Source: CAD feature listing. Evaluate the final solid. Frame: model axes, mm. Face numbers are marked on the shaded views. Round coordinates to 2 decimals unless told otherwise and drop trailing zeros. Order: outer loops, then holes, each group sorted by start corner. A loop starts at its lowest first (then second) coordinate and runs counter-clockwise, first axis right, second up. Notation, with made-up numbers: M -6,28 L 50,28 A25 cw 50,41 Z; hole C 50,-7.75 d7. An arc over 180 degrees is marked long. Use one line per item in the form item = value. Start each with the question number.
Q1. Section A-A (x = 29.8). Give the number of separate pieces and of enclosed holes in the cut face, plus the area to 3 significant figures.
Q2. Section D-D (x = 25.5). Return the cut outline in (y, z), plus the area to 3 significant figures.
Q3. Pull-direction query (Y, two-part tool) for the marked faces 1, 2 and 3; classes: pulls with the +Y half, pulls with the -Y half, needs draft (parallel to the pull), parting line crosses it, or undercut.
Q4. Section C-C (z = 7). Return the cut outline in (x, y).
Q5. Contact query for flat-ended pins moving along their axis: pin 1 (4.5 mm diameter, centred on x = 29.8, y = 9.8, fed in from +Z); pin 2 (5 mm diameter, centred on x = 30, y = 10.5, fed in from +Z); pin 3 (6 mm diameter, centred on x = 35, y = 12, fed in from +Z). Output: stop coordinate, or through.
Q6. Material intervals for probe 1 along Y at (x, z) = (9.8, 4.25); probe 2 along Y at (x, z) = (29.8, 0.85); probe 3 along Y at (x, z) = (5.5, 8), sorted ascending.
from build123d import *

# Parameters (mm, degrees)
SKETCH_W        = 39.6
SKETCH_H        = 39.6
PAD_DEPTH       = 9
SKETCH001_R     = 1.75
POCKET_DEPTH    = 10
SKETCH002_R     = 3
POCKET001_DEPTH = 6
SKETCH003_W     = 30
SKETCH003_H     = 30
POCKET002_DEPTH = 3
FILLET_R        = 1


with BuildPart() as part:
    # Sketch → Pad (new body)
    with BuildSketch(Plane.XY):
        with Locations((19.8, 19.8)):
            Rectangle(SKETCH_W, SKETCH_H)
    extrude(amount=PAD_DEPTH)

    # Sketch001 → Pocket (cut)
    with BuildSketch(Plane.XY.offset(9)):
        with Locations((9.8, 9.8)):
            Circle(SKETCH001_R)
        with Locations((9.8, 29.8)):
            Circle(SKETCH001_R)
        with Locations((29.8, 9.8)):
            Circle(SKETCH001_R)
        with Locations((29.8, 29.8)):
            Circle(SKETCH001_R)
    extrude(amount=-POCKET_DEPTH, mode=Mode.SUBTRACT)

    # Sketch002 → Pocket001 (cut)
    with BuildSketch(Plane.XY.offset(9)):
        with Locations((9.8, 9.8)):
            Circle(SKETCH002_R)
        with Locations((9.8, 29.8)):
            Circle(SKETCH002_R)
        with Locations((29.8, 9.8)):
            Circle(SKETCH002_R)
        with Locations((29.8, 29.8)):
            Circle(SKETCH002_R)
    extrude(amount=-POCKET001_DEPTH, mode=Mode.SUBTRACT)

    # Sketch003 → Pocket002 (cut)
    with BuildSketch(Plane.XY.offset(9)):
        with Locations((19.8, 19.8)):
            Rectangle(SKETCH003_W, SKETCH003_H)
    extrude(amount=-POCKET002_DEPTH, mode=Mode.SUBTRACT)

    # Fillet
    fillet_edges = [part.edges().sort_by_distance(p)[0] for p in [
        (0, 39.6, 4.5),
        (0, 0, 4.5),
        (39.6, 39.6, 4.5),
        (39.6, 0, 4.5),
        (39.6, 19.8, 0),
        (19.8, 39.6, 0),
        (0, 19.8, 0),
        (19.8, 0, 0),
        (19.8, 0, 9),
        (39.6, 19.8, 9),
        (19.8, 39.6, 9),
        (0, 19.8, 9),
        (19.8, 4.8, 9),
        (34.8, 19.8, 9),
        (19.8, 34.8, 9),
        (4.8, 19.8, 9),
    ]]
    fillet(fillet_edges, radius=FILLET_R)


solid = part.part
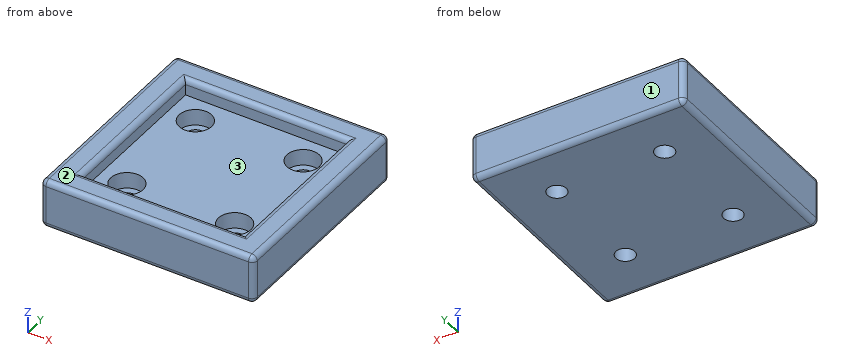
Results list:
q1.separate_pieces = 3
q1.enclosed_holes = 0
q1.area = 208 mm2
q2.outline = M 0,1 A1 ccw 1,0 L 38.6,0 A1 ccw 39.6,1 L 39.6,8 A1 ccw 38.6,9 L 35.8,9 A1 ccw 34.8,8 L 34.8,6 L 4.8,6 L 4.8,8 A1 ccw 3.8,9 L 1,9 A1 ccw 0,8 Z
q2.area = 265 mm2
q3.face_1 = pulls with the +Y half
q3.face_2 = needs draft
q3.face_3 = undercut
q4.outline = M 0,1 A1 ccw 1,0 L 38.6,0 A1 ccw 39.6,1 L 39.6,38.6 A1 ccw 38.6,39.6 L 1,39.6 A1 ccw 0,38.6 Z; hole M 4.8,4.8 L 34.8,4.8 L 34.8,34.8 L 4.8,34.8 Z
q5.pin_1 = 3
q5.pin_2 = 6
q5.pin_3 = 9
q6.probe_1 = 0 to 6.8, 12.8 to 26.8, 32.8 to 39.6
q6.probe_2 = 0.01 to 8.05, 11.55 to 28.05, 31.55 to 39.59
q6.probe_3 = 0 to 4.8, 34.8 to 39.6
